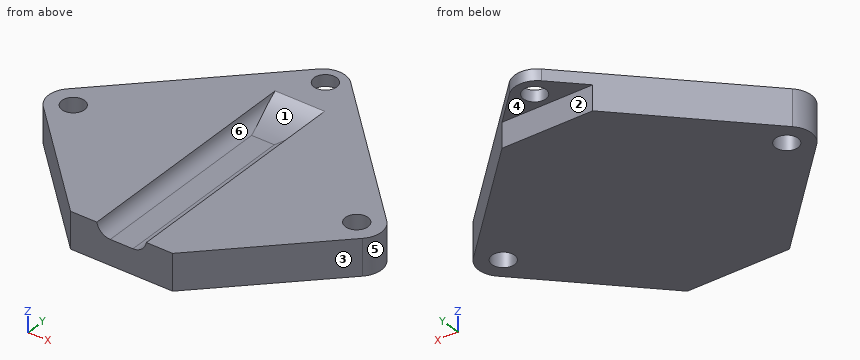
```python
from build123d import *

# Parameters (mm, degrees)
SKETCH1_R           = 1
BOSS_EXTRUDE1_DEPTH = 3.2
CUT_EXTRUDE1_DEPTH  = 21
FILLET1_R           = 10
CUT_EXTRUDE3_DEPTH  = 2.2


with BuildPart() as part:
    # Sketch1 → Boss-Extrude1 (new body)
    with BuildSketch(Plane.XY):
        with BuildLine():
            Line((-13.537758799, -2.661648107), (-3.951972362, -12.247434544))
            Line((-3.951972362, -12.247434544), (5.048027638, -12.247434544))
            Line((5.048027638, -12.247434544), (14.633814076, -2.661648107))
            ThreePointArc((14.633814076, -2.661648107), (15.219600513, -1.247434544), (14.633814076, 0.166779018))
            Line((14.633814076, 0.166779018), (1.962241201, 12.838351893))
            ThreePointArc((1.962241201, 12.838351893), (0.548027638, 13.424138331), (-0.866185924, 12.838351893))
            Line((-0.866185924, 12.838351893), (-13.537758799, 0.166779018))
            ThreePointArc((-13.537758799, 0.166779018), (-14.123545237, -1.247434544), (-13.537758799, -2.661648107))
        make_face()
        with Locations((-11.951972362, -1.247434544)):
            Circle(SKETCH1_R, mode=Mode.SUBTRACT)
        with Locations((13.048027638, -1.247434544)):
            Circle(SKETCH1_R, mode=Mode.SUBTRACT)
        with Locations((0.548027638, 11.752565456)):
            Circle(SKETCH1_R, mode=Mode.SUBTRACT)
    extrude(amount=BOSS_EXTRUDE1_DEPTH)

    # Sketch2 → Cut-Extrude1 (cut)
    with BuildSketch(Plane.XZ.offset(12.247434544)):
        with BuildLine():
            Line((-0.451972362, 4.603907064), (1.548027638, 4.603907064))
            ThreePointArc((1.548027638, 4.603907064), (2.748027638, 3.403907064), (1.548027638, 2.203907064))
            Line((1.548027638, 2.203907064), (-0.451972362, 2.203907064))
            ThreePointArc((-0.451972362, 2.203907064), (-1.651972362, 3.403907064), (-0.451972362, 4.603907064))
        make_face()
    extrude(amount=-CUT_EXTRUDE1_DEPTH, mode=Mode.SUBTRACT)

    # Fillet1
    # the kernel refuses this fillet: 10 mm, written as the material it adds along each edge
    with BuildSketch(Plane(origin=(12.425084222, 8.752565456, 2.203907064), x_dir=(0, -1, 0), z_dir=(-1, 0, 0))) as fillet1_piece_1_section:
        with BuildLine():
            CenterArc((4.350822634, 10), FILLET1_R, 244.209471462, 25.790528538)
            Line((0, 0.996092936), (0, 0))
            Line((0, 0), (4.350822634, 0))
        make_face()
    fillet1_piece_1 = extrude(amount=23.754113168, mode=Mode.PRIVATE)
    fillet1_piece_1 = split(fillet1_piece_1, bisect_by=Plane(origin=(-2.713667021, 10.990870796, 2.436615037), z_dir=(0.7071067811865476, -0.7071067811865475, 0)), keep=Keep.TOP, mode=Mode.PRIVATE)
    fillet1_piece_1 = split(fillet1_piece_1, bisect_by=Plane(origin=(4.900996749, 9.899596345, 2.436615037), z_dir=(-0.7071067811865476, -0.7071067811865476, 0)), keep=Keep.TOP, mode=Mode.PRIVATE)
    add(fillet1_piece_1)

    # Sketch5 → Cut-Extrude3 (cut)
    with BuildSketch(Plane(origin=(0, 0, 0), x_dir=(-1, 0, 0), z_dir=(0, 0, -1))):
        Polygon((-4.548027638, 10.252565456), (-0.548027638, 14.252565456), (3.451972362, 10.252565456), align=None)
    extrude(amount=-CUT_EXTRUDE3_DEPTH, mode=Mode.SUBTRACT)


solid = part.part
```
The model under review builds one solid part; all positions refer to its coordinate system, in mm. Face numbers are marked on the shaded views. A direction names the side the tool comes from. Round coordinates to 2 decimals unless told otherwise and drop trailing zeros. Write each loop counter-clockwise with the first axis right and the second up, starting at its lowest first coordinate (ties: lowest second). Pieces come first, ordered by that corner, then holes. Notation, with made-up numbers: (17, 79.5) - (73, 79.5) arc R19 ccw to (73, 88.5) - close; hole circle Ø9 at (30.25, 57.25). An arc over 180 degrees is marked (long way). Use one line per item in the form item = value.
Q1. Consider section D-D (y = -10). State the section outline as (x, z) points.
Answer key:
outline = (-6.2, 0) - (7.3, 0) - (7.3, 3.2) - (2.73, 3.2) arc R1.2 cw to (1.55, 2.2) - (-0.45, 2.2) arc R1.2 cw to (-1.63, 3.2) - (-6.2, 3.2) - close
Q2. Tool access review of the marked faces 1, 2 and 3: name each direction out of +Z, -Z, +X, -X, +Y, -Y from which nothing blocks a thin tool from reaching the whole face with its end or side.
Answer key:
face_1 = +Z, -Y
face_2 = -Z, +X, -X, +Y
face_3 = +Z, -Z, +X, -Y
Q3. Draft analysis for pull direction X (two halves, no side actions). For the marked faces 4, 5 and 6, state which applies: +X half, -X half, draft (parallel to the pull), parting line (faces both ways), or undercut.
Answer key:
face_4 = draft
face_5 = +X half
face_6 = undercut
Q4. Consider section A-A (z = 0.55). State the section outline as (x, y) points.
Answer key:
outline = (-13.54, -2.66) - (-3.95, -12.25) - (5.05, -12.25) - (14.63, -2.66) arc R2 ccw to (14.63, 0.17) - (4.55, 10.25) - (-3.45, 10.25) - (-13.54, 0.17) arc R2 ccw to start; hole circle Ø2 at (-11.95, -1.25); hole circle Ø2 at (13.05, -1.25)
Q5. Consider section C-C (x = -8.5). State the section outline as (y, z) points, and give its area (3 significant figures).
Answer key:
outline = (-7.7, 0) - (5.2, 0) - (5.2, 3.2) - (-7.7, 3.2) - close
area = 41.3 mm2
Q6. Consider section B-B (y = -6). State the section outline as (x, z) points, and give its area (3 significant figures).
Answer key:
outline = (-10.2, 0) - (11.3, 0) - (11.3, 3.2) - (2.73, 3.2) arc R1.2 cw to (1.55, 2.2) - (-0.45, 2.2) arc R1.2 cw to (-1.63, 3.2) - (-10.2, 3.2) - close
area = 65.0 mm2
Q7. Insertion check: pin 1 Ø10 at (x, y) = (-1.5, 2) entering from -Z; pin 2 Ø1 at (x, y) = (1, -6.5) entering from +Z; pin 3 Ø6 at (x, y) = (-10.5, 9.5) entering from +Z; pin 4 Ø1.8 at (x, z) = (1.5, 1.5) entering from +Y. Each pin has a flat end and moves straight along its axis. Give the tip position at first contact, or say it passes through.
Answer key:
pin_1 = 0
pin_2 = 2.2
pin_3 = through
pin_4 = 13.39
Q8. For line 1 (Y direction, x = 4.5, z = 1.75); line 2 (Y direction, x = -12.5, z = 1.4); line 3 (X direction, y = -8, z = 2.35), list the stretches that pass through material, from the lowest coordinate up. Write a range as [from, to].
Answer key:
line_1 = [-12.25, 10.25]
line_2 = [-3.7, -2.08], [-0.41, 1.2]
line_3 = [-8.2, -1.03], [2.12, 9.3]
